Geometry check sheet. Reference: the model listing, model coordinates, mm. Round coordinates to 2 decimals unless told otherwise and drop trailing zeros. Write each loop counter-clockwise with the first axis right and the second up, starting at its lowest first coordinate (ties: lowest second). Pieces come first, ordered by that corner, then holes. Notation, with made-up numbers: M 56,75.5 L 70,75.5 A32 ccw 70,109.5 Z; hole C 24,11.5 d8. An arc over 180 degrees is marked long. Use a Markdown table: item, result.
```python
from build123d import *

# Parameters (mm, degrees)
SKETCH1_W           = 14
SKETCH1_H           = 7
BOSS_EXTRUDE1_DEPTH = 204
CUT_EXTRUDE1_DEPTH  = 8
CUT_EXTRUDE2_DEPTH  = 8


with BuildPart() as part:
    # Sketch1 → Boss-Extrude1 (new body)
    with BuildSketch(Plane.XY):
        with Locations((7, 3.5)):
            Rectangle(SKETCH1_W, SKETCH1_H)
    extrude(amount=BOSS_EXTRUDE1_DEPTH)

    # Sketch2 → Cut-Extrude1 (cut, through all)
    with BuildSketch(Plane(origin=(0, 7, 0), x_dir=(1, 0, 0), z_dir=(0, 1, 0))):
        Polygon((0, 0), (14, -14), (14, 0), align=None)
        Polygon((14, -204), (0, -204), (14, -190), align=None)
    extrude(amount=-CUT_EXTRUDE1_DEPTH, mode=Mode.SUBTRACT)

    # Sketch3 → Cut-Extrude2 (cut, through all)
    with BuildSketch(Plane(origin=(0, 7, 0), x_dir=(1, 0, 0), z_dir=(0, 1, 0))):
        with BuildLine():
            Line((8.272792206, -195.727207794), (5.727207794, -198.272792206))
            ThreePointArc((5.727207794, -198.272792206), (5.727207794, -195.727207794), (8.272792206, -195.727207794))
        make_face()
        with BuildLine():
            Line((5.727207794, -5.727207794), (8.272792206, -8.272792206))
            ThreePointArc((8.272792206, -8.272792206), (5.727207794, -8.272792206), (5.727207794, -5.727207794))
        make_face()
    extrude(amount=-CUT_EXTRUDE2_DEPTH, mode=Mode.SUBTRACT)


solid = part.part
```
Item 1: Material ranges on line 1 along Z through (x, y) = (5.5, 4); line 2 along Z through (x, y) = (4.5, 6); line 3 along Z through (x, y) = (7.75, 5), recorded low to high. Write a range as from..to.
Outcome:
| item | result |
|---|---|
| line 1 | z = 5.5..6.01, 7.99..196.01, 197.99..198.5 |
| line 2 | z = 4.5..199.5 |
| line 3 | z = 8.64..195.36 |
Item 2: Mould release check, pull along X, two halves, no side actions. Record for faces 1 (the face through (7, 0, 101)), 2 (the face through (11, 4, 193)), 3 (the face through (0, 3, 101)), 4 (the face through (5.7, 3.549, 195.756)): +X half, -X half, draft (parallel to the pull), parting line (faces both ways), or undercut.
Outcome:
| item | result |
|---|---|
| face 1 | draft |
| face 2 | +X half |
| face 3 | -X half |
| face 4 | undercut |
Item 3: Cross-section at A-A, the plane y = 2.75. Record the cut outline in (x, z).
Outcome:
| item | result |
|---|---|
| outline | M 0,0 L 5.73,5.73 A1.8 cw 8.27,8.27 L 14,14 L 14,190 L 8.27,195.73 A1.8 cw 5.73,198.27 L 0,204 Z |
Item 4: Go/stop test with flat-tipped pins: pin 1 (1 mm diameter, centred on x = 11, y = 4.5, fed in from -Z); pin 2 (2 mm diameter, centred on x = 11, y = 2.5, fed in from -Z); pin 3 (4 mm diameter, centred on x = 3.5, y = 3.5, fed in from +Z). Record where each tip stops, or that it passes through.
Outcome:
| item | result |
|---|---|
| pin 1 | stops at z = 10.5 |
| pin 2 | stops at z = 10 |
| pin 3 | stops at z = 202.5 |
Item 5: Cross-section at B-B, the plane x = 2.75. Record the cut outline in (y, z), and give its area (3 significant figures).
Outcome:
| item | result |
|---|---|
| outline | M 0,2.75 L 7,2.75 L 7,201.25 L 0,201.25 Z |
| area | 1,390 mm2 |
